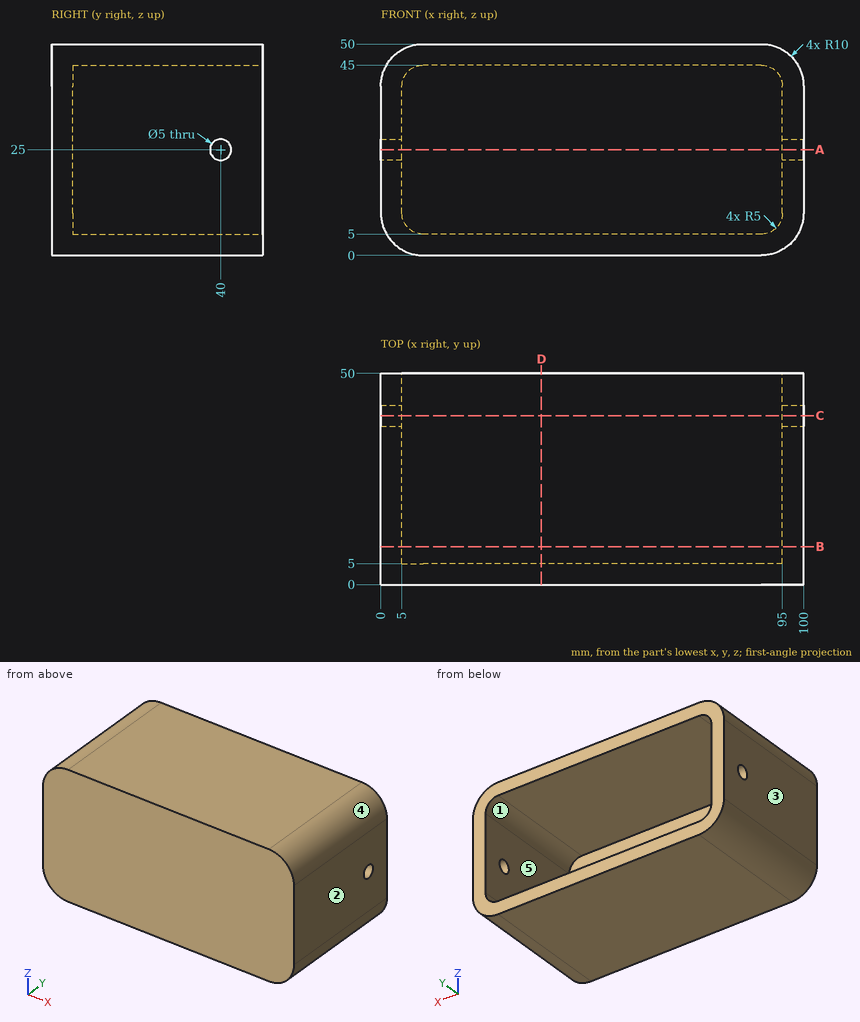
Study the drawing (mm; zero at the part's minimum x, y, z) and answer. A direction names the side the tool comes from. Give positions to 0.01 mm unless a question says otherwise; leave off trailing zeros. Loops run counter-clockwise (first coordinate to the right, second up) from the corner with the lowest first, then second, coordinate; pieces in that order, holes last. Notation, with made-up numbers: (-17, 6.25) - (32, 6.25) arc R9 ccw to (32, 22.25) - close; hole circle Ø4 at (55.25, -19). An arc over 180 degrees is marked (long way). Answer in a Markdown table with one row per item. Add a question column.
Q1. A tool of negligible diameter and unlimited length cuts with its end or side. For the marked faces 4 and 5, from which of +Z, -Z, +X, -X, +Y, -Y can it reach the whole face along a straight path? Write none if from no direction.
Q2. The part is cut by section C-C (y = 40). Determine the outline of the cut face in (x, z).
Q3. Determine the mould class of the marked faces 1, 2 and 3 for opening direction X: released by +X, released by -X, zero draft, split by the parting line, or undercut.
Q4. The part is cut by section B-B (y = 9). Determine the outline of the cut face in (x, z).
Q5. The part is cut by section A-A (z = 25). Determine the outline of the cut face in (x, y).
Q6. Consider line 1 along X through (y, z) = (12, 18); line 2 along Y through (x, z) = (98.5, 25); line 3 along Z through (x, y) = (66.5, 28). Determine where each line is inside the solid, lowest interval first.
Q7. Each of these flat-tipped pins is pushed along its axis until it touches: P1, Ø3, axis at y = 20.5, z = 7, coming from the -X side; P2, Ø5, axis at x = 34.5, z = 22, coming from the +Y side; P3, Ø1.5, axis at y = 37.5, z = 44, coming from the -X side. Where does it stop, or does it pass through?
Q8. The part is cut by section D-D (x = 38). Determine the outline of the cut face in (y, z).
Solution:
| question | item | result |
|---|---|---|
| 1 | face 4 | +Z, +X, +Y, -Y |
| 1 | face 5 | +Y |
| 2 | outline | (0, 10) arc R10 ccw to (10, 0) - (90, 0) arc R10 ccw to (100, 10) - (100, 22.5) - (95, 22.5) - (95, 10) arc R5 cw to (90, 5) - (10, 5) arc R5 cw to (5, 10) - (5, 22.5) - (0, 22.5) - close; (0, 27.5) - (5, 27.5) - (5, 40) arc R5 cw to (10, 45) - (90, 45) arc R5 cw to (95, 40) - (95, 27.5) - (100, 27.5) - (100, 40) arc R10 ccw to (90, 50) - (10, 50) arc R10 ccw to (0, 40) - close |
| 3 | face 1 | undercut |
| 3 | face 2 | released by +X |
| 3 | face 3 | released by -X |
| 4 | outline | (0, 10) arc R10 ccw to (10, 0) - (90, 0) arc R10 ccw to (100, 10) - (100, 40) arc R10 ccw to (90, 50) - (10, 50) arc R10 ccw to (0, 40) - close; hole (5, 10) arc R5 ccw to (10, 5) - (90, 5) arc R5 ccw to (95, 10) - (95, 40) arc R5 ccw to (90, 45) - (10, 45) arc R5 ccw to (5, 40) - close |
| 5 | outline | (0, 0) - (100, 0) - (100, 37.5) - (95, 37.5) - (95, 5) - (5, 5) - (5, 37.5) - (0, 37.5) - close; (0, 42.5) - (5, 42.5) - (5, 50) - (0, 50) - close; (95, 42.5) - (100, 42.5) - (100, 50) - (95, 50) - close |
| 6 | line 1 | x = 0 to 5, 95 to 100 |
| 6 | line 2 | y = 0 to 37.5, 42.5 to 50 |
| 6 | line 3 | z = 0 to 5, 45 to 50 |
| 7 | P1 | stops at x = 0.11 |
| 7 | P2 | stops at y = 5 |
| 7 | P3 | stops at x = 0.54 |
| 8 | outline | (0, 0) - (50, 0) - (50, 5) - (5, 5) - (5, 45) - (50, 45) - (50, 50) - (0, 50) - close |
